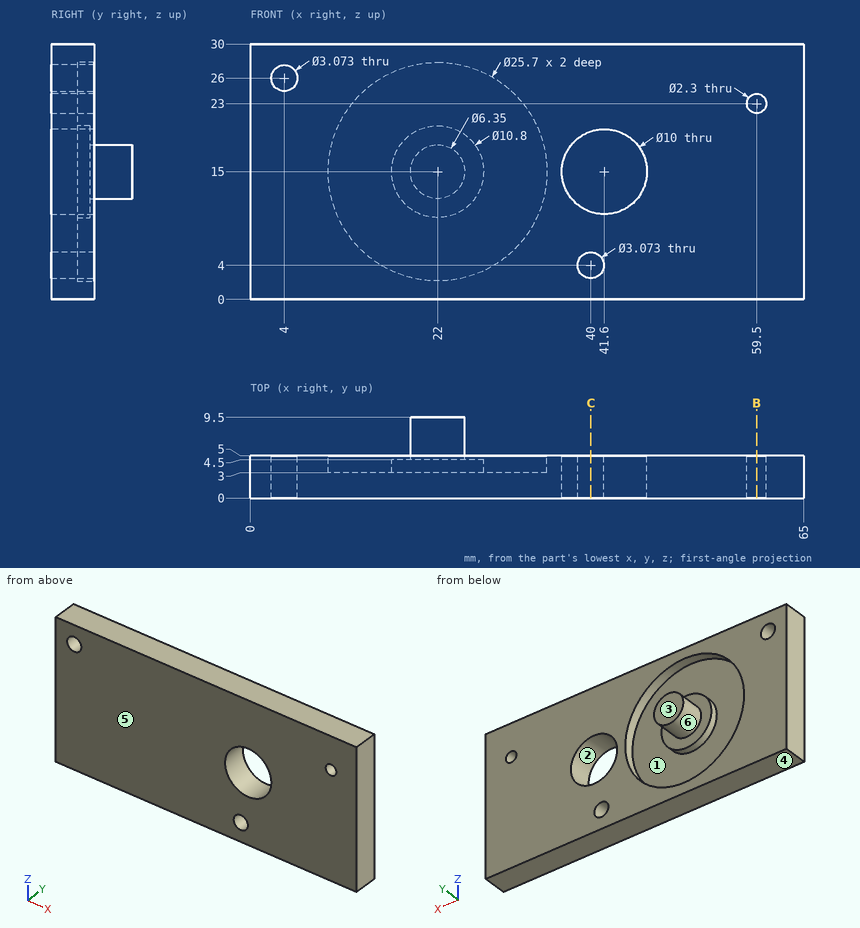
Study the drawing (mm; zero at the part's minimum x, y, z) and answer. A direction names the side the tool comes from. Give positions to 0.01 mm unless a question says otherwise; leave off trailing zeros. Write each loop counter-clockwise with the first axis right and the second up, starting at its lowest first coordinate (ties: lowest second). Pieces come first, ordered by that corner, then holes. Notation, with made-up numbers: (61, 72.25) -> (113, 72.25) arc R14 cw to (113, 82.25) -> close; hole circle Ø7 at (86.25, -22.5). An arc over 180 degrees is marked (long way). Answer as a JSON object with one key per item and string values. Group by question number.
1) A tool of negligible diameter and unlimited length cuts with its end or side. For the marked faces 5 and 6, from which of +Z, -Z, +X, -X, +Y, -Y can it reach the whole face along a straight path? Write none if from no direction.
2) Consider L1, parallel to X at y = 3.8, z = 15; L2, parallel to X at y = 4, z = 18.75 (1 decimal); L3, parallel to Y at x = 32, z = 7.5. Determine where each line is inside the solid, lowest interval first. Write a range as from..to.
3) Each of these flat-tipped pins is pushed along its axis until it touches: P1, Ø12, axis at x = 54, z = 17, coming from the +Y side; P2, Ø2, axis at x = 16, z = 12.5, coming from the +Y side; P3, Ø2.5, axis at x = 40, z = 4, coming from the -Y side; P4, Ø4, axis at y = 8.5, z = 15, coming from the +X side (3 decimals). Where does it stop, or does it pass through?
4) Find section B-B (x = 59.5). Write down the section's boundary in (y, z).
5) The mould has two halves that part along Z. Classify the marked faces 1, 2, 3 and 4: +Z half, -Z half, draft (parallel to the pull), parting line (faces both ways), or undercut.
6) Find section C-C (x = 40). Write down the section's boundary in (y, z).
Values follow:
{
 "1": {"face 5": "+Z, -Z, +X, -X, -Y", "face 6": "+Y"},
 "2": {"L1": "x = 0..9.15, 16.6..27.4, 34.85..36.6, 46.6..65", "L2": "x = 0..9.7, 18.1..25.9, 34.3..38.3, 44.9..65", "L3": "y = 0..3"},
 "3": {"P1": "stops at y = 5", "P2": "stops at y = 3", "P3": "passes through", "P4": "stops at x = 25.175"},
 "4": {"outline": "(0, 0) -> (5, 0) -> (5, 21.85) -> (0, 21.85) -> close; (0, 24.15) -> (5, 24.15) -> (5, 30) -> (0, 30) -> close"},
 "5": {"face 1": "undercut", "face 2": "undercut", "face 3": "draft", "face 4": "-Z half"},
 "6": {"outline": "(0, 0) -> (5, 0) -> (5, 2.46) -> (0, 2.46) -> close; (0, 5.54) -> (5, 5.54) -> (5, 10.26) -> (0, 10.26) -> close; (0, 19.74) -> (5, 19.74) -> (5, 30) -> (0, 30) -> close"}
}
